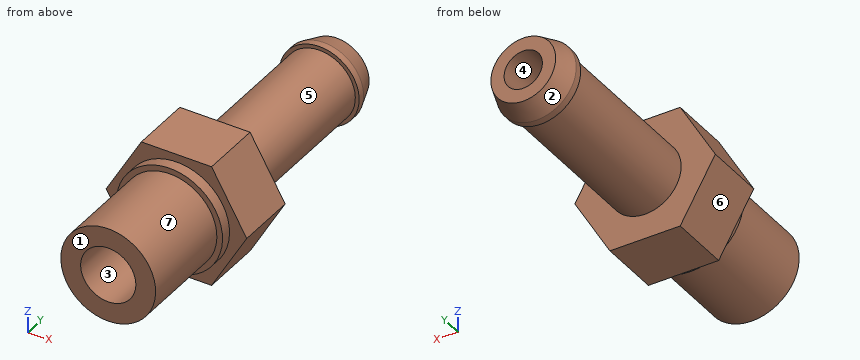
from build123d import *

# Parameters (mm, degrees)
BOSS_EXTRUDE1_DEPTH = 8.0391
SKETCH3_R           = 4.7371
BOSS_EXTRUDE2_DEPTH = 21.8059
SKETCH4_R           = 5.23875
BOSS_EXTRUDE3_DEPTH = 0.9271
SKETCH11_R          = 6.96595
BOSS_EXTRUDE4_DEPTH = 1.4605
SKETCH12_R          = 6.223
BOSS_EXTRUDE5_DEPTH = 12.8016
SKETCH24_R          = 2.5146
CUT_EXTRUDE1_DEPTH  = 50.298716199
SKETCH25_R          = 3.62585
CUT_EXTRUDE2_DEPTH  = 16.4592


with BuildPart() as part:
    # Sketch1 → Boss-Extrude1 (new body)
    with BuildSketch(Plane(origin=(0, 0, 0), x_dir=(1, 0, 0), z_dir=(0, 1, 0))):
        Polygon((9.224094311, 0), (4.612047155, 7.9883), (-4.612047155, 7.9883), (-9.224094311, 0), (-4.612047155, -7.9883), (4.612047155, -7.9883), align=None)
    extrude(amount=BOSS_EXTRUDE1_DEPTH)

    # Sketch3 → Boss-Extrude2 (add)
    with BuildSketch(Plane(origin=(0, 8.0391, 0), x_dir=(1, 0, 0), z_dir=(0, 1, 0))):
        with Locations(Location((0, 0, 0), (0, 0, 270))):
            Circle(SKETCH3_R)
    extrude(amount=BOSS_EXTRUDE2_DEPTH)

    # Sketch4 → Boss-Extrude3 (add)
    with BuildSketch(Plane(origin=(0, 29.845, 0), x_dir=(1, 0, 0), z_dir=(0, 1, 0))):
        with Locations(Location((0, 0, 0), (0, 0, 270))):
            Circle(SKETCH4_R)
    extrude(amount=BOSS_EXTRUDE3_DEPTH)

    # Sketch10 → Revolve1 (revolve)
    with BuildSketch(Plane(origin=(0, 0, 0), x_dir=(0, 0, -1), z_dir=(1, 0, 0)), mode=Mode.PRIVATE) as revolve1_sk:
        Polygon((0, 30.7721), (0, 33.5026), (-2.49555, 33.5026), (-4.2545, 33.5026), (-5.23875, 30.7721), align=None)
    revolve(revolve1_sk.sketch.rotate(Axis((0, 30.7721, 0), (0, 1, 0)), 180), axis=Axis((0, 30.7721, 0), (0, 1, 0)))

    # Sketch11 → Boss-Extrude4 (add)
    with BuildSketch(Plane(origin=(0, 0, 0), x_dir=(-1, 0, 0), z_dir=(0, -1, 0))):
        with Locations(Location((0, 0, 0), (0, 0, 90))):
            Circle(SKETCH11_R)
    extrude(amount=BOSS_EXTRUDE4_DEPTH)

    # Sketch12 → Boss-Extrude5 (add)
    with BuildSketch(Plane(origin=(0, -1.4605, 0), x_dir=(-1, 0, 0), z_dir=(0, -1, 0))):
        with Locations(Location((0, 0, 0), (0, 0, 90))):
            Circle(SKETCH12_R)
    extrude(amount=BOSS_EXTRUDE5_DEPTH)

    # Sketch24 → Cut-Extrude1 (cut, through all)
    with BuildSketch(Plane(origin=(0, 33.5026, 0), x_dir=(1, 0, 0), z_dir=(0, 1, 0))):
        with Locations(Location((0, 0, 0), (0, 0, 270))):
            Circle(SKETCH24_R)
    extrude(amount=-CUT_EXTRUDE1_DEPTH, mode=Mode.SUBTRACT)

    # Sketch25 → Cut-Extrude2 (cut)
    with BuildSketch(Plane(origin=(0, -14.2621, 0), x_dir=(-1, 0, 0), z_dir=(0, -1, 0))):
        with Locations(Location((0, 0, 0), (0, 0, 90))):
            Circle(SKETCH25_R)
    extrude(amount=-CUT_EXTRUDE2_DEPTH, mode=Mode.SUBTRACT)


solid = part.part
Input: part model. Units: mm. Frame: model coordinates. Face numbers are marked on the shaded views. A direction names the side the tool comes from. Round coordinates to 2 decimals unless told otherwise and drop trailing zeros. Write each loop counter-clockwise with the first axis right and the second up, starting at its lowest first coordinate (ties: lowest second). Pieces come first, ordered by that corner, then holes.
1) Reachability of the marked faces 5, 6 and 7 from +Z, -Z, +X, -X, +Y, -Y: full face, straight path, thin tool, end or side. Return the list, or none.
2) Cut plane B-B (x = 7.75). Return the cut outline in (y, z), then the cut area to 3 significant figures.
3) Cut plane A-A (y = 4). Return the cut outline in (x, z).
4) Cut plane C-C (y = 12). Return the cut outline in (x, z).
5) Contact query for flat-ended pins moving along their axis: P1, Ø1, axis at y = -4, z = 5, coming from the -X side; P2, Ø8.5, axis at x = 0, z = 0, coming from the -Y side; P3, Ø1, axis at x = 0, y = 14, coming from the +Z side; P4, Ø4, axis at x = -0.5, y = 27.5, coming from the -Z side. Output: stop coordinate, or through.
6) Ray query, L1, parallel to X at y = 27, z = 0; L2, parallel to X at y = -7.75, z = 0; L3, parallel to Y at x = -5, z = 3.75. Return the intervals inside material, ascending.
7) Draft query along X for the marked faces 1, 2, 3 and 4. Return one class per face: pulls with the +X half, pulls with the -X half, needs draft (parallel to the pull), parting line crosses it, or undercut.
Geometry says:
1. face 5: none
1. face 6: -Z, -X, +Y, -Y
1. face 7: -Y
2. outline: (0, -2.55) - (8.04, -2.55) - (8.04, 2.55) - (0, 2.55) - close
2. area: 41.1 mm2
3. outline: (-9.22, 0) - (-4.61, -7.99) - (4.61, -7.99) - (9.22, 0) - (4.61, 7.99) - (-4.61, 7.99) - close; hole circle Ø5.03 at (0, 0)
4. outline: circle Ø9.47 at (0, 0); hole circle Ø5.03 at (0, 0)
5. P1: stops at x = -4.3
5. P2: stops at y = -14.26
5. P3: stops at z = 4.74
5. P4: stops at z = -4.74
6. L1: x = -4.74 to -2.51, 2.51 to 4.74
6. L2: x = -6.22 to -3.63, 3.63 to 6.22
6. L3: y = -1.46 to 8.04
7. face 1: needs draft
7. face 2: parting line crosses it
7. face 3: undercut
7. face 4: undercut
